from build123d import *

# Parameters (mm, degrees)
SKETCH2_R           = 5
BOSS_EXTRUDE1_DEPTH = 150
CHAMFER1_SIZE       = 1


with BuildPart() as part:
    # Sketch1 → Revolve1 (revolve)
    with BuildSketch(Plane.XY, mode=Mode.PRIVATE) as revolve1_sk:
        Polygon((0, 0), (0, 302), (4, 302), (5, 301), (5, 1), (4, 0), align=None)
    revolve(revolve1_sk.sketch.rotate(Axis((0, 0, 0), (0, 1, 0)), 90), axis=Axis((0, 0, 0), (0, 1, 0)))

    # Sketch2 → Boss-Extrude1 (add, symmetric)
    with BuildSketch(Plane.XY):
        Circle(SKETCH2_R)
    extrude(amount=BOSS_EXTRUDE1_DEPTH, both=True)

    # Chamfer1
    chamfer1_edges = [part.edges().sort_by_distance(p)[0] for p in [
        (-5, 0, -150),
        (-5, 0, 150),
    ]]
    chamfer(chamfer1_edges, length=CHAMFER1_SIZE)


solid = part.part
The listing builds one solid part. Answer for the finished solid, in the listing's coordinates (mm). A direction names the side the tool comes from. Coordinates: 2 decimals unless noted, no trailing zeros. Write each loop counter-clockwise with the first axis right and the second up, starting at its lowest first coordinate (ties: lowest second). Pieces come first, ordered by that corner, then holes. Notation, with made-up numbers: M 88,34 L 137,34 A20 ccw 137,42 Z; hole C 59,15 d11. An arc over 180 degrees is marked long. Put each result on its own line as item: value. Start each with the question number.
1. A cutting plane is placed at B-B on z = 65.5. Write down the section's boundary in (x, y).
2. Which of the six approach directions +Z, -Z, +X, -X, +Y, -Y give full straight-line access (tool end or side, diameter ignored) to faces 1 (the cylindrical face through (0, 149, 5)), 2 (the cylindrical face through (-1.08, -4.88, 2.09)), 3 (the flat face through (0, 0, 150))?
3. A cutting plane is placed at A-A on x = 0. Write down the section's boundary in (y, z).
4. Flat-ended cylindrical pins translate along their axes: P1, Ø2, axis at x = -2.5, z = -62.5, coming from the +Y side; P2, Ø1.5, axis at x = 3, y = 38, coming from the -Z side. Find the tip coordinate at first contact, or state that the pin passes through.
5. Consider line 1 (Y direction, x = -1.25, z = -83); line 2 (Y direction, x = 1, z = 80); line 3 (Z direction, x = 0.75, y = 107). Determine where each line is inside the solid, lowest interval first. Write a range as from..to.
Resolved:
1. outline: C 0,0 d10
2. face 1: +Y
2. face 2: none
2. face 3: +Z, +X, -X, +Y, -Y
3. outline: M -5,-149 L -4,-150 L 4,-150 L 5,-149 L 5,-5 L 301,-5 L 302,-4 L 302,4 L 301,5 L 5,5 L 5,149 L 4,150 L -4,150 L -5,149 Z
4. P1: stops at y = 4.77
4. P2: stops at z = -4.47
5. line 1: y = -4.84..4.84
5. line 2: y = -4.9..4.9
5. line 3: z = -4.94..4.94
